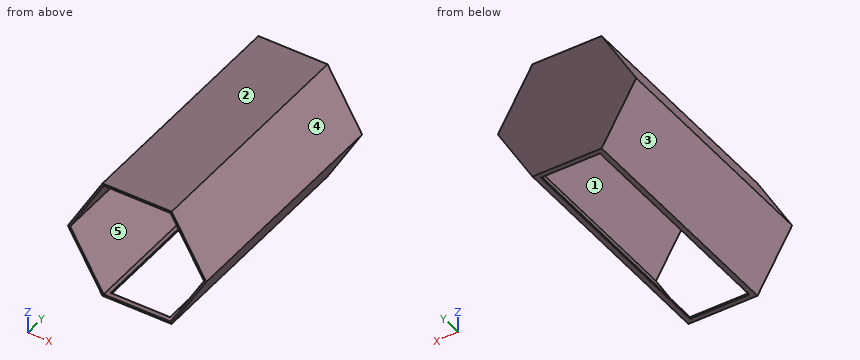
Autodesk Fusion 360 part; units mm, degrees
sketch "side" plane through (0, 0, 0) normal (0, 1, 0) x (1, 0, 0)
  line L0 (35, -60.6218) -> (70, 0)
  line L1 (70, 0) -> (35, 60.6218)
  line L2 (35, 60.6218) -> (-35, 60.6218)
  line L3 (-35, 60.6218) -> (-70, 0)
  line L4 (-70, 0) -> (-35, -60.6218)
  line L5 (-35, -60.6218) -> (35, -60.6218)
  dimension "d1" = 70
extrude "Extrude1" add sketch "side" along normal blind 240
sketch "2mm offset cap" plane through (0, 0, 0) normal (0, -1, 0) x (1, 0, 0)
  line L0 (35, 60.6218) -> (-35, 60.6218)
  line L1 (-35, 60.6218) -> (-70, 0)
  line L2 (-70, 0) -> (-35, -60.6218)
  line L3 (-35, -60.6218) -> (35, -60.6218)
  line L4 (35, -60.6218) -> (70, 0)
  line L5 (70, 0) -> (35, 60.6218)
  line L6 (-35, 60.6218) -> (35, 60.6218)
  line L7 (70, 0) -> (35, 60.6218)
  line L8 (70, 0) -> (35, -60.6218)
  line L9 (35, -60.6218) -> (-35, -60.6218)
  line L10 (-35, -60.6218) -> (-70, 0)
  line L11 (-70, 0) -> (-35, 60.6218)
  line L12 (-33.8453, -58.6218) -> (-67.6906, 0)
  line L13 (-67.6906, 0) -> (-33.8453, 58.6218)
  line L14 (-33.8453, 58.6218) -> (33.8453, 58.6218)
  line L15 (67.6906, 0) -> (33.8453, 58.6218)
  line L16 (67.6906, 0) -> (33.8453, -58.6218)
  line L17 (33.8453, -58.6218) -> (-33.8453, -58.6218)
  dimension "d4" = 2
extrude "Extrude2" cut sketch "2mm offset cap" against normal blind 239 contours L12 L13 L14 L15 L16 L17
sketch "opening for tubes" plane through (0, 0, -60.6218) normal (0, 0, -1) x (1, 0, 0)
  line L0 (35, 0) -> (-35, 0)
  line L1 (-35, 0) -> (-35, -240)
  line L2 (-35, -240) -> (35, -240)
  line L3 (35, -240) -> (35, 0)
  line L4 (-35, -240) -> (35, -240)
  line L5 (35, -240) -> (35, 0)
  line L6 (35, 0) -> (-35, 0)
  line L7 (-35, 0) -> (-35, -240)
  line L8 (30, -235) -> (30, -5)
  line L9 (30, -5) -> (-30, -5)
  line L10 (-30, -5) -> (-30, -235)
  line L11 (-30, -235) -> (30, -235)
  dimension "d7" = -5
extrude "Extrude4" cut sketch "opening for tubes" against normal blind 2 contours L8 L9 L10 L11
Read the model definition and answer for the solid it produces. Units are mm, in the model's axes. Face numbers are marked on the shaded views. A direction names the side the tool comes from. Give positions to 0.01 mm unless a question says otherwise; leave off trailing zeros. Write each loop counter-clockwise with the first axis right and the second up, starting at its lowest first coordinate (ties: lowest second). Pieces come first, ordered by that corner, then holes. Notation, with made-up numbers: (25, 63) - (33, 63) arc R17 cw to (33, 67) - close; hole circle Ø8 at (84, 16.5). An arc over 180 degrees is marked (long way). Use CSV: the item, a comma, the result in double quotes. Start each with the question number.
(1) Find section A-A (x = 6). Give the vertices of the cut face in (y, z), plus the area to 3 significant figures.
(2) Find section D-D (x = 38.5). Give the vertices of the cut face in (y, z), plus the area to 3 significant figures.
(3) Given P1, Ø3, axis at y = 46, z = 2, coming from the +X side; P2, Ø6, axis at y = 102, z = 26, coming from the +X side; P3, Ø2, axis at y = 154, z = -59.5, coming from the +X side (3 decimals), each flat-ended and moving along its own axis, determine where each tip first touches the part or whether it passes through.
(4) Consider line 1 along Z through (x, y) = (16.5, 14); line 2 along Z through (x, y) = (53, 101); line 3 along Z through (x, y) = (33, 54). Determine where each line is inside the solid, lowest interval first.
(5) Determine the mould class of the marked faces 1, 2 and 3 for opening direction Z: +Z half, -Z half, draft (parallel to the pull), parting line (faces both ways), or undercut.
(6) Find section C-C (z = -37). Give the vertices of the cut face in (x, y), plus the area to 3 significant figures.
(7) For the marked faces 4 and 5, determine the directions among +Z, -Z, +X, -X, +Y, -Y from which every point of the face is accessible in a straight line to the end or side of a thin tool.
(8) Find section B-B (y = 225.5). Give the vertices of the cut face in (x, z), plus the area to 3 significant figures.
Findings below:
1,outline,"(0, -60.62) - (5, -60.62) - (5, -58.62) - (0, -58.62) - close; (0, 58.62) - (239, 58.62) - (239, -58.62) - (235, -58.62) - (235, -60.62) - (240, -60.62) - (240, 60.62) - (0, 60.62) - close"
1,area,"617 mm2"
2,outline,"(0, -54.56) - (240, -54.56) - (240, 54.56) - (0, 54.56) - (0, 50.56) - (239, 50.56) - (239, -50.56) - (0, -50.56) - close"
2,area,"2,020 mm2"
3,P1,"x = 69.71"
3,P2,"x = 56.72"
3,P3,"x = 36.225"
4,line 1,"58.62 to 60.62"
4,line 2,"-29.44 to -25.44, 25.44 to 29.44"
4,line 3,"-60.62 to -58.62, 58.62 to 60.62"
5,face 1,"undercut"
5,face 2,"+Z half"
5,face 3,"-Z half"
6,outline,"(-48.64, 0) - (-46.33, 0) - (-46.33, 239) - (46.33, 239) - (46.33, 0) - (48.64, 0) - (48.64, 240) - (-48.64, 240) - close"
6,area,"1,200 mm2"
7,face 4,"+Z, +X, +Y, -Y"
7,face 5,"-Y"
8,outline,"(-70, 0) - (-35, -60.62) - (-30, -60.62) - (-30, -58.62) - (-33.85, -58.62) - (-67.69, 0) - (-33.85, 58.62) - (33.85, 58.62) - (67.69, 0) - (33.85, -58.62) - (30, -58.62) - (30, -60.62) - (35, -60.62) - (70, 0) - (35, 60.62) - (-35, 60.62) - close"
8,area,"706 mm2"
